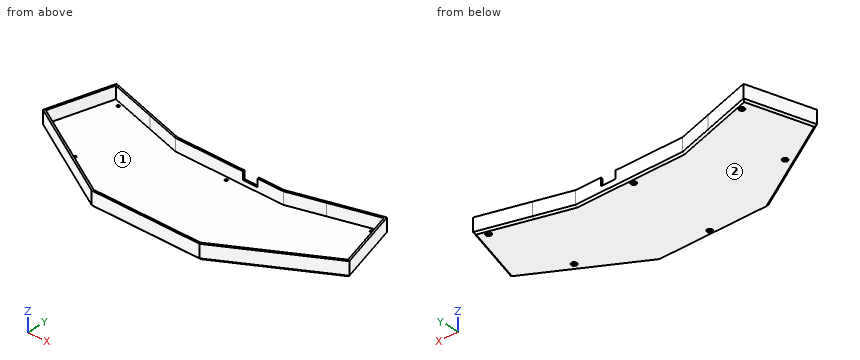
from build123d import *

# Parameters (mm, degrees)
BOSS_EXTRU_1_DEPTH      = 14
BOSS_EXTRU_2_DEPTH      = 3
ENL_V_START             = 5
ENL_V_MAT_EXTRU_1_DEPTH = 10
ESQUISSE7_R             = 1.5
ENL_V_MAT_EXTRU_2_DEPTH = 10
ESQUISSE8_R             = 3
ENL_V_MAT_EXTRU_3_DEPTH = 2
CHANFREIN1_SIZE         = 2


with BuildPart() as part:
    # Esquisse1 → Boss.-Extru.1 (new body)
    with BuildSketch(Plane.XY):
        Polygon((229.15721289, -14.84723942), (106.433306853, -14.84723942), (67.372523259, -3.649091023), (12.961214213, 11.953100779), (-7.58450021, -59.698320459), (106.05278448, -124.898736851), (229.537735263, -124.898736851), (343.175019953, -59.698320459), (322.62930553, 11.953100779), (268.217996484, -3.649091023), align=None)
        Polygon((229.438237844, -16.84723942), (106.152281899, -16.84723942), (66.821302011, -5.571629745), (14.332462893, 9.479302675), (-5.230075099, -58.743374877), (106.585792597, -122.898736851), (229.004727146, -122.898736851), (340.820594842, -58.743374877), (321.25805685, 9.479302675), (268.769217732, -5.571629745), align=None, mode=Mode.SUBTRACT)
    extrude(amount=BOSS_EXTRU_1_DEPTH)

    # Esquisse2 → Boss.-Extru.2 (add)
    with BuildSketch(Plane(origin=(0, 0, 0), x_dir=(-1, 0, 0), z_dir=(0, 0, -1))):
        Polygon((-229.15721289, -14.84723942), (-268.217996484, -3.649091023), (-322.62930553, 11.953100779), (-343.175019953, -59.698320459), (-229.537735263, -124.898736851), (-106.05278448, -124.898736851), (7.58450021, -59.698320459), (-12.961214213, 11.953100779), (-67.372523259, -3.649091023), (-106.433306853, -14.84723942), align=None)
    extrude(amount=BOSS_EXTRU_2_DEPTH)

    # Esquisse3 → Enlèv. mat.-Extru.1 (cut)
    with BuildSketch(Plane.XY.offset(ENL_V_START)):
        Polygon((193.384025698, 6.988548589), (218.304917235, -79.922959834), (202.924702789, -84.333062282), (178.003811253, 2.578446141), align=None)
    extrude(amount=ENL_V_MAT_EXTRU_1_DEPTH, mode=Mode.SUBTRACT)

    # Esquisse7 → Enlèv. mat.-Extru.2 (cut)
    with BuildSketch(Plane.XY):
        with Locations((312.747989314, 2.877882334)):
            Circle(ESQUISSE7_R)
        with Locations((167.795259872, -20.84723942)):
            Circle(ESQUISSE7_R)
        with Locations(Location((22.842530429, 2.877882334, 0), (0, 0, 180))):
            Circle(ESQUISSE7_R)
        with Locations(Location((167.795259872, -118.898736851, 0), (0, 0, 180))):
            Circle(ESQUISSE7_R)
        with Locations((46.946880967, -80.077290604)):
            Circle(ESQUISSE7_R)
        with Locations(Location((288.643638776, -80.077290604, 0), (0, 0, 180))):
            Circle(ESQUISSE7_R)
    extrude(amount=-ENL_V_MAT_EXTRU_2_DEPTH, mode=Mode.SUBTRACT)

    # Esquisse8 → Enlèv. mat.-Extru.3 (cut)
    with BuildSketch(Plane(origin=(0, 0, -3), x_dir=(-1, 0, 0), z_dir=(0, 0, -1))):
        with Locations((-22.842530429, 2.877882334)):
            Circle(ESQUISSE8_R)
        with Locations((-46.946880967, -80.077290604)):
            Circle(ESQUISSE8_R)
        with Locations((-167.795259872, -118.898736851)):
            Circle(ESQUISSE8_R)
        with Locations((-167.795259872, -20.84723942)):
            Circle(ESQUISSE8_R)
        with Locations((-288.643638776, -80.077290604)):
            Circle(ESQUISSE8_R)
        with Locations((-312.747989314, 2.877882334)):
            Circle(ESQUISSE8_R)
    extrude(amount=-ENL_V_MAT_EXTRU_3_DEPTH, mode=Mode.SUBTRACT)

    # Chanfrein1
    chanfrein1_edges = [part.edges().sort_by_distance(p)[0] for p in [
        (167.795259872, -14.84723942, -3),
        (248.687604687, -9.248165222, -3),
        (295.423651007, 4.152004878, -3),
        (332.902162742, -23.87260984, -3),
        (286.356377608, -92.298528655, -3),
        (167.795259872, -124.898736851, -3),
        (49.234142135, -92.298528655, -3),
        (2.688357001, -23.87260984, -3),
        (40.166868736, 4.152004878, -3),
        (86.902915056, -9.248165222, -3),
    ]]
    chamfer(chanfrein1_edges, length=CHANFREIN1_SIZE)


solid = part.part
Geometry: final body of the model. Coordinates: model frame, mm. Face numbers are marked on the shaded views. Coordinates: 2 decimals unless noted, no trailing zeros. Order: outer loops, then holes, each group sorted by start corner. A loop starts at its lowest first (then second) coordinate and runs counter-clockwise, first axis right, second up.
(1) Section query C-C (y = -37). Return the cut outline in (x, z), plus the area to 3 significant figures.
(2) First-contact query: pin 1 (1.8 mm diameter, centred on x = 311.5, y = 3.5, fed in from -Z); pin 2 (10 mm diameter, centred on y = -45.5, z = 3.5, fed in from +X); pin 3 (3 mm diameter, centred on x = 176, z = 5, fed in from +Y); pin 4 (7 mm diameter, centred on x = 312.75, y = 2.88, fed in from -Z). Flat tips, straight axial feed; report the tip coordinate or a pass-through.
(3) Draft query along X for the marked faces 1 and 2. Return one class per face: pulls with the +X half, pulls with the -X half, needs draft (parallel to the pull), parting line crosses it, or undercut.
(4) Section query A-A (z = 9.75). Return the cut outline in (x, y), plus the area to 3 significant figures.
(5) Section query B-B (x = 127.5). Return the cut outline in (y, z).
(6) Material intervals for probe 1 along Y at (x, z) = (144, 12.5); probe 2 along Z at (x, y) = (254, -78.5); probe 3 along X at (y, z) = (-37, 1), sorted ascending.
Solution:
1. outline: (-1.08, -1) - (1, -3) - (334.59, -3) - (336.67, -1) - (336.67, 14) - (334.59, 14) - (334.59, 0) - (1, 0) - (1, 14) - (-1.08, 14) - close
1. area: 1,070 mm2
2. pin 1: stops at z = -1
2. pin 2: stops at x = 340.54
2. pin 3: stops at y = -14.85
2. pin 4: stops at z = -3
3. face 1: undercut
3. face 2: needs draft
4. outline: (-7.58, -59.7) - (106.05, -124.9) - (229.54, -124.9) - (343.18, -59.7) - (322.63, 11.95) - (268.22, -3.65) - (229.16, -14.85) - (199.65, -14.85) - (200.22, -16.85) - (229.44, -16.85) - (268.77, -5.57) - (321.26, 9.48) - (340.82, -58.74) - (229, -122.9) - (106.59, -122.9) - (-5.23, -58.74) - (14.33, 9.48) - (66.82, -5.57) - (106.15, -16.85) - (183.57, -16.85) - (183, -14.85) - (106.43, -14.85) - (67.37, -3.65) - (12.96, 11.95) - close
4. area: 1,660 mm2
5. outline: (-124.9, -1) - (-122.9, -3) - (-16.85, -3) - (-14.85, -1) - (-14.85, 14) - (-16.85, 14) - (-16.85, 0) - (-122.9, 0) - (-122.9, 14) - (-124.9, 14) - close
6. probe 1: y = -124.9 to -122.9, -16.85 to -14.85
6. probe 2: z = -3 to 0
6. probe 3: x = -1.08 to 1, 334.59 to 336.67
